Geometry check sheet. Reference: the model listing, model coordinates, mm. A direction names the side the tool comes from. Round coordinates to 2 decimals unless told otherwise and drop trailing zeros. Order: outer loops, then holes, each group sorted by start corner. A loop starts at its lowest first (then second) coordinate and runs counter-clockwise, first axis right, second up. Notation, with made-up numbers: M 73,-11 L 95,-11 A31 cw 95,13 Z; hole C 56.5,16 d11. An arc over 180 degrees is marked long. Answer as a JSON object with one key per item and string values. Group by question number.
Autodesk Inventor part; units mm, degrees
ref_plane "Work Plane1" through (17.8247, 6, -6.6364) normal (0, 0, 1) x (1, 0, 0)
ref_plane "YZ Plane" through (0, 0, 0) normal (1, 0, 0) x (0, 1, 0)
ref_plane "XZ Plane" through (0, 0, 0) normal (0, 1, 0) x (-1, 0, 0)
sketch "Sketch1" plane through (0, 0, 0) normal (0, 1, 0) x (-1, 0, 0)
  line L0 (16.1753, 16.3636) -> (-28.8247, 16.3636)
  line L1 (-28.8247, 16.3636) -> (-28.8247, 6.3636)
  line L2 (16.1753, 6.3636) -> (16.1753, 16.3636)
  line L3 (-17.8247, 6.3636) -> (-17.8247, 1.3636)
  line L4 (-17.8247, 1.3636) -> (5.1753, 1.3636)
  line L5 (5.1753, 1.3636) -> (5.1753, 6.3636)
  line L6 (-28.8247, 6.3636) -> (-17.8247, 6.3636)
  line L7 (5.1753, 6.3636) -> (16.1753, 6.3636)
  point P0 (0, 0)
  dimension "d4" = 45
  dimension "d5" = 5
  dimension "d6" = 5
  dimension "d7" = 11
  dimension "d8" = 11
  dimension "d9" = 23
  dimension "d10" = 10
extrude "Extrusion1" add sketch "Sketch1" along normal blind 6
sketch "Sketch4" plane through (17.8247, 0, 6.3636) normal (1, 0, 0) x (0, 0, -1)
  circle A0 centre (7, 6) radius 6
  line L0 (0, 6) -> (5, 6)
  line L1 (0, 0) -> (0, 6)
  point P0 (6.3636, 0)
  dimension "d20" = 12
  dimension "d21" = 0
  dimension "d36" = 7
extrude "Extrusion4" add sketch "Sketch4" against normal up to surface (23 mm away)
fillet "Fillet1" radius 12 2 edges at (6.3247, 0.3431, 1.3636) (6.3247, 0, 1.3636)
sketch "Sketch5" plane through (17.8247, 0, 6.3636) normal (1, 0, 0) x (0, 0, -1)
  circle A0 centre (7, 6) radius 6
  circle A1 centre (7, 6) radius 2.5
  point P0 (6.3636, 0)
  point P1 (1, 6)
  point P2 (6.25, 0.0471)
  dimension "d27" = 5
extrude "Extrusion5" cut sketch "Sketch5" against normal through all contours A1
ref_plane "Work Plane1" through (17.8247, 6, -6.6364) normal (0, 0, 1) x (1, 0, 0)
sketch "Sketch6" plane through (0, 6, 0) normal (0, 1, 0) x (1, 0, 0)
  circle A0 centre (-9.0753, -11.1636) radius 2.5
  circle A1 centre (21.7247, -11.1636) radius 2.5
  line L0 (37.8247, 6.6364) -> (-25.1753, 6.6364)
  line L1 (28.8247, -16.3636) -> (28.8247, -6.3636)
  line L2 (-16.1753, -6.3636) -> (-16.1753, -16.3636)
  point P0 (0, 0)
  dimension "d33" = 5
  dimension "d34" = 5
  dimension "d35" = 17.8
  dimension "d37" = 17.8
  dimension "d38" = 7.1
  dimension "d39" = 30.8
  dimension "d40" = 7.1
extrude "Extrusion6" cut sketch "Sketch6" against normal through all
move faces "Move1" translate (-2.5, 0, 0) faces at (17.8247, 3.6127, 3.7179)
move faces "Move2" translate (2.5, 0, 0) faces at (-5.1753, 3.6127, 3.7179) (1.658, 5.7988, -3.1283)
properties part number "Cerniera 1"
1) Go/stop test with flat-tipped pins: P1, Ø12, axis at x = 0, z = 12.5, coming from the +Y side; P2, Ø6, axis at y = 6.5, z = 2, coming from the +X side; P3, Ø1.8, axis at x = 25, y = 2.5, coming from the -Z side. Record where each tip stops, or that it passes through.
2) Sectioned sample at A-A (y = 4.75). Record the boundary of the cut face in (x, z).
3) Release check for a two-part mould opening along Z. For faces 1 (the flat face through (-9, 3, 6.364)), 2 (the flat face through (6, 3, 16.364)), 3 (the flat face through (15.325, 3, 0)), 4 (the cylindrical face through (-6.69, 3.04, 10.41)) record: +Z half, -Z half, draft (parallel to the pull), parting line (faces both ways), or undercut.
4) Sectioned sample at B-B (x = 3). Record the boundary of the cut face in (y, z).
5) Set-up check for faces 5 (the flat face through (7, 6, 11)), 6 (the cylindrical face through (24.034, 3.042, 12.121)), 7 (the flat face through (-2.675, 3, 0)), 8 (the flat face through (28.825, 3, 11)), 9 (the flat face through (22, 3, 6.364)): record each of +Z, -Z, +X, -X, +Y, -Y from which the full face is reachable in a straight line by a thin tool's end or side.
6) Thickness scan on line 1 along X through (y, z) = (5.25, 10.25); line 2 along X through (y, z) = (5.75, 12.25); line 3 along Y through (x, z) = (9.5, -0.5). Record the ranges inside material, lowest first. Write a range as [from, to].
7) Sectioned sample at C-C (z = 12.75). Record the boundary of the cut face in (x, y).
Final values:
{
 "1": {"P1": "stops at y = 6", "P2": "stops at x = 15.32", "P3": "stops at z = 6.36"},
 "2": {"outline": "M -16.18,6.36 L -2.68,6.36 L -2.68,1.53 L 15.32,1.53 L 15.32,6.36 L 28.82,6.36 L 28.82,16.36 L -16.18,16.36 Z; M -2.68,-6.5 L 15.32,-6.5 L 15.32,-2.8 L -2.68,-2.8 Z; hole C -9.08,11.16 d5; hole C 21.72,11.16 d5"},
 "3": {"face 1": "-Z half", "face 2": "+Z half", "face 3": "draft", "face 4": "undercut"},
 "4": {"outline": "M 0,4.21 A12 ccw 0.07,2.91 A12 cw 0.05,0.11 A6 ccw long 6,5.36 L 6,16.36 L 0,16.36 Z; hole C 6,-0.64 d5"},
 "5": {"face 5": "+Z, +X, -X, +Y", "face 6": "+Y, -Y", "face 7": "-Z, -X, +Y, -Y", "face 8": "+Z, -Z, +X, +Y, -Y", "face 9": "-Z, +X, +Y, -Y"},
 "6": {"line 1": "x = [-16.18, -11.4], [-6.75, 19.4], [24.05, 28.82]", "line 2": "x = [-16.18, -11.33], [-6.82, 19.47], [23.98, 28.82]", "line 3": "y = [0, 3.5], [8.5, 12]"},
 "7": {"outline": "M -16.18,0 L -11.01,0 L -11.01,6 L -16.18,6 Z; M -7.14,0 L 19.79,0 L 19.79,6 L -7.14,6 Z; M 23.66,0 L 28.82,0 L 28.82,6 L 23.66,6 Z"}
}
